Part model, mm, in its own coordinate system. A direction names the side the tool comes from. Give positions to 0.01 mm unless a question says otherwise; leave off trailing zeros. Order: outer loops, then holes, each group sorted by start corner. A loop starts at its lowest first (then second) coordinate and runs counter-clockwise, first axis right, second up.
1. Slice it at A-A on y = 39.5. List the corners of the cut face in (x, z).
2. Slice it at B-B on z = 62. List the corners of the cut face in (x, y).
3. Which spindle directions (+Z, -Z, +X, -X, +Y, -Y) get a long thin tool onto all of the face, cutting with end or side? Do faces 4 (the flat face through (88, 24, 911.86)), 5 (the flat face through (88, 26, 0)). Say none if no direction does.
4. Probe line 1 (X direction, y = 25, z = 913); line 2 (Z direction, x = 92, y = 42); line 3 (X direction, y = 9, z = 402). List the from-to ranges inside material, lowest first.
5. Drop flat-ended pins along their axis: pin 1 Ø4 at (x, y) = (55.5, 18) entering from -Z; pin 2 Ø8 at (x, z) = (30.5, 192.5) entering from -Y. Give the stop position or say it passes through.
6. Slice it at C-C on x = 152.5. List the corners of the cut face in (y, z), and give its area (3 significant figures).
7. Mould opens along X. For faces 1 (the flat face through (88, 26, 914.4)), 2 (the flat face through (0, 25, 451)), 3 (the flat face through (88, 48.26, 451)) say: +X half, -X half, draft (parallel to the pull), parting line (faces both ways), or undercut.
from build123d import *

# Parameters (mm, degrees)
SKETCH1_W           = 177.8
SKETCH1_H           = 50.8
BOSS_EXTRUDE1_DEPTH = 914.4
SHELL1_T            = -2.54
SKETCH2_R           = 3.175
CUT_EXTRUDE1_DEPTH  = 945.134


with BuildPart() as part:
    # Sketch1 → Boss-Extrude1 (new body)
    with BuildSketch(Plane.XY):
        with Locations((88.9, 25.4)):
            Rectangle(SKETCH1_W, SKETCH1_H)
    extrude(amount=BOSS_EXTRUDE1_DEPTH)

    # Shell1
    shell1_openings = [part.faces().sort_by_distance(p)[0] for p in [
        (88.9, 0, 457.2),
    ]]
    offset(amount=SHELL1_T, openings=shell1_openings, kind=Kind.INTERSECTION)

    # Sketch2 → Cut-Extrude1 (cut)
    with BuildSketch(Plane(origin=(0, 0, 0), x_dir=(-1, 0, 0), z_dir=(0, 0, -1))):
        with Locations((-44.45, 25.4)):
            Circle(SKETCH2_R)
        with Locations((-133.35, 25.4)):
            Circle(SKETCH2_R)
    extrude(amount=-CUT_EXTRUDE1_DEPTH, mode=Mode.SUBTRACT)


solid = part.part
Data:
1. outline: (0, 0) - (177.8, 0) - (177.8, 914.4) - (0, 914.4) - close; hole (2.54, 2.54) - (175.26, 2.54) - (175.26, 911.86) - (2.54, 911.86) - close
2. outline: (0, 0) - (2.54, 0) - (2.54, 48.26) - (175.26, 48.26) - (175.26, 0) - (177.8, 0) - (177.8, 50.8) - (0, 50.8) - close
3. face 4: -Y
3. face 5: -Z, +X, -X, +Y, -Y
4. line 1: x = 0 to 41.3, 47.6 to 130.2, 136.5 to 177.8
4. line 2: z = 0 to 2.54, 911.86 to 914.4
4. line 3: x = 0 to 2.54, 175.26 to 177.8
5. pin 1: stops at z = 0
5. pin 2: stops at y = 48.26
6. outline: (0, 0) - (50.8, 0) - (50.8, 914.4) - (0, 914.4) - (0, 911.86) - (48.26, 911.86) - (48.26, 2.54) - (0, 2.54) - close
6. area: 2,570 mm2
7. face 1: draft
7. face 2: -X half
7. face 3: undercut
